```python
from build123d import *

# Parameters (mm, degrees)
SKETCH1_R                = 1.6
SKETCH1_R_2              = 6.45
BOSS_EXTRUDE1_DEPTH      = 3.175
SKETCH4_R                = 1.675
BOSS_EXTRUDE3_DEPTH      = 6.25
SKETCH4_2_R              = 1.675
CUT_EXTRUDE2_DEPTH       = 2.63125
FILLET1_R                = 2
FILLET2_R                = 2
FILLET3_R                = 2
CIRPATTERN2_COUNT        = 3
FILLET1_OF_CIRPATTERN2_R = 2
FILLET2_OF_CIRPATTERN2_R = 2
FILLET3_OF_CIRPATTERN2_R = 2
FILLET5_R                = 0.75


with BuildPart() as part:
    # Sketch1 → Boss-Extrude1 (new body)
    with BuildSketch(Plane.XY):
        with BuildLine():
            Line((15.347308801, 31.210973101), (8.051491314, 33.998880179))
            ThreePointArc((8.051491314, 33.998880179), (5.696175566, 34.15336703), (3.663829908, 32.952971436))
            Line((3.663829908, 32.952971436), (-1.653149933, 27.103867562))
            ThreePointArc((-1.653149933, 27.103867562), (-2.154824203, 26.417727613), (-2.500196213, 25.641078866))
            Line((-2.500196213, 25.641078866), (-9.325438013, 4.478720632))
            ThreePointArc((-9.325438013, 4.478720632), (-9.502063256, 3.613546149), (-9.484560317, 2.730700176))
            Line((-9.484560317, 2.730700176), (-8.507421128, -4.718687488))
            ThreePointArc((-8.507421128, -4.718687488), (-7.54564448, -6.839386894), (-5.565731281, -8.065080174))
            Line((-5.565731281, -8.065080174), (2.031002829, -10.077591551))
            ThreePointArc((2.031002829, -10.077591551), (2.960636861, -10.209852347), (3.895489669, -10.121746843))
            Line((3.895489669, -10.121746843), (25.485057009, -5.483666514))
            ThreePointArc((25.485057009, -5.483666514), (26.373611638, -5.180049941), (27.166902489, -4.677653705))
            Line((27.166902489, -4.677653705), (33.329625608, 0.328323939))
            ThreePointArc((33.329625608, 0.328323939), (34.614533997, 2.205289229), (34.668387555, 4.479291881))
            Line((34.668387555, 4.479291881), (32.591741985, 12.142614371))
            ThreePointArc((32.591741985, 12.142614371), (32.241466178, 13.013831458), (31.697738169, 13.779384986))
            Line((31.697738169, 13.779384986), (16.88625911, 30.157458595))
            ThreePointArc((16.88625911, 30.157458595), (16.17904213, 30.77516119), (15.347308801, 31.210973101))
        make_face()
        with Locations((24.879793107, 5.344918551)):
            Circle(SKETCH1_R, mode=Mode.SUBTRACT)
        with Locations((7.811061307, 24.218992148)):
            Circle(SKETCH1_R, mode=Mode.SUBTRACT)
        Circle(SKETCH1_R, mode=Mode.SUBTRACT)
        with Locations((10.896951472, 9.8546369)):
            Circle(SKETCH1_R_2, mode=Mode.SUBTRACT)
    extrude(amount=BOSS_EXTRUDE1_DEPTH)

    # Sketch4 → Boss-Extrude3 (add, symmetric)
    with BuildSketch(Plane(origin=(0.449621982, -0.475334512, 0), x_dir=(-0.726482741, -0.687184711, 0), z_dir=(0.687184711, -0.726482741, 0))):
        Polygon((-31.72132028, 0), (-31.72132028, -3.175), (-25.539496086, -3.175), (-31.72132028, -5.425), (-41.88132028, -5.425), (-41.88132028, 0), align=None)
        with Locations((-36.80132028, -2.7125)):
            Circle(SKETCH4_R, mode=Mode.SUBTRACT)
    boss_extrude3 = extrude(amount=BOSS_EXTRUDE3_DEPTH, both=True)

    # Sketch4<2> → Cut-Extrude2 (cut, symmetric)
    with BuildSketch(Plane(origin=(0.449621982, -0.475334512, 0), x_dir=(-0.726482741, -0.687184711, 0), z_dir=(0.687184711, -0.726482741, 0))):
        Polygon((-31.72132028, 0), (-31.72132028, -3.175), (-25.539496086, -3.175), (-31.72132028, -5.425), (-41.88132028, -5.425), (-41.88132028, 0), align=None)
        with Locations((-36.80132028, -2.7125)):
            Circle(SKETCH4_2_R, mode=Mode.SUBTRACT)
    cut_extrude2 = extrude(amount=CUT_EXTRUDE2_DEPTH, both=True, mode=Mode.SUBTRACT)

    # Fillet1
    fillet1_edges = [part.edges().sort_by_distance(p)[0] for p in [
        (19.440964609, 21.110601986, 3.175),
        (23.057274153, 17.287486564, 3.175),
        (25.865326768, 14.96244967, 3.175),
        (17.377217607, 24.139682361, 3.175),
        (22.0551547, 13.848979318, 3.175),
        (15.952095481, 20.301054157, 3.175),
    ]]
    fillet(fillet1_edges, radius=FILLET1_R)

    # Fillet2
    fillet2_edges = [part.edges().sort_by_distance(p)[0] for p in [
        (25.302768444, 19.411514101, 1.5875),
        (21.6864589, 23.234629523, 1.5875),
    ]]
    fillet(fillet2_edges, radius=FILLET2_R)

    # Fillet3
    fillet3_edges = [part.edges().sort_by_distance(p)[0] for p in [
        (27.824148706, 31.530905901, 0),
        (33.927207925, 25.078831062, 0),
        (33.927207925, 25.078831062, 5.425),
        (27.824148706, 31.530905901, 5.425),
    ]]
    fillet(fillet3_edges, radius=FILLET3_R)

    # CirPattern2: Boss-Extrude3, Cut-Extrude2 ×3 about axis
    cirpattern2_axis = Axis((10.896951472, 9.8546369, 0), (0, 0, 1))
    for i in range(1, CIRPATTERN2_COUNT):
        add(boss_extrude3.rotate(cirpattern2_axis, i * 360 / CIRPATTERN2_COUNT))
        add(cut_extrude2.rotate(cirpattern2_axis, i * 360 / CIRPATTERN2_COUNT), mode=Mode.SUBTRACT)

    # Fillet1 of CirPattern2
    fillet1_of_cirpattern2_edges = [part.edges().sort_by_distance(p)[0] for p in [
        (-3.123006806, 11.625986784, 3.175),
        (-1.620246501, 16.669360428, 3.175),
        (-1.010731793, 20.263723774, 3.175),
        (-4.71439386, 8.324189266, 3.175),
        (1.858647852, 17.520753147, 3.175),
        (-0.677483256, 9.009311403, 3.175),
        (16.372896612, -3.172678071, 3.175),
        (11.253826762, -4.392936293, 3.175),
        (7.836259441, -5.662262745, 3.175),
        (20.028030667, -2.899960928, 3.175),
        (8.777051863, -1.805821766, 3.175),
        (17.41624219, 0.253545139, 3.175),
    ]]
    fillet(fillet1_of_cirpattern2_edges, radius=FILLET1_OF_CIRPATTERN2_R)

    # Fillet2 of CirPattern2
    fillet2_of_cirpattern2_edges = [part.edges().sort_by_distance(p)[0] for p in [
        (-4.582455452, 17.552001759, 1.5875),
        (-6.085215757, 12.508628115, 1.5875),
        (11.970541423, -7.399605162, 1.5875),
        (17.089611272, -6.17934694, 1.5875),
    ]]
    fillet(fillet2_of_cirpattern2_edges, radius=FILLET2_OF_CIRPATTERN2_R)

    # Fillet3 of CirPattern2
    fillet3_of_cirpattern2_edges = [part.edges().sort_by_distance(p)[0] for p in [
        (-16.33884676, 13.675885219, 0),
        (-13.802715652, 22.187326963, 0),
        (-13.802715652, 22.187326963, 5.425),
        (-16.33884676, 13.675885219, 5.425),
        (21.205552469, -15.642880421, 0),
        (12.566362141, -17.702247326, 0),
        (12.566362141, -17.702247326, 5.425),
        (21.205552469, -15.642880421, 5.425),
    ]]
    fillet(fillet3_of_cirpattern2_edges, radius=FILLET3_OF_CIRPATTERN2_R)

    # Fillet5
    fillet5_edges = [part.edges().sort_by_distance(p)[0] for p in [
        (-7.789671487, 9.240521362, 1.5875),
        (-3.951849266, 21.140080535, 1.5875),
        (20.879758905, -6.473021336, 1.5875),
        (8.655527257, -9.099149384, 1.5875),
        (20.045714571, 26.663830856, 2.5875),
        (28.432123998, 17.390399731, 2.5875),
    ]]
    fillet(fillet5_edges, radius=FILLET5_R)


solid = part.part
```
The listing builds one solid part. Answer for the finished solid, in the listing's coordinates (mm). A direction names the side the tool comes from. Round coordinates to 2 decimals unless told otherwise and drop trailing zeros. Use one line per item in the form item = value. Start each with the question number.
1. Given pin 1 Ø3 at (x, y) = (8, -12) entering from +Z (3 decimals); pin 2 Ø4 at (x, y) = (0, 0) entering from +Z (3 decimals); pin 3 Ø2 at (x, z) = (-5, 4.5) entering from -Y; pin 4 Ø3 at (x, z) = (0, 1.5) entering from -Y, each flat-ended and moving along its own axis, determine where each tip first touches the part or whether it passes through.
2. For a pull along X with two mould halves and no side action, classify faces 6 (the face through (23.53, -5.904, 1.775)), 7 (the face through (10.06, 16.25, 1.57)), 8 (the face through (11, -12, 5.425)) as pulls with the +X half, pulls with the -X half, needs draft (parallel to the pull), parting line crosses it, or undercut.
3. Consider line 1 (Z direction, x = 1.5, y = 15) (3 decimals); line 2 (X direction, y = 8.5, z = 2.7); line 3 (X direction, y = 25, z = 2.7). Determine where each line is inside the solid, lowest interval first. Write a range as [from, to].
4. A tool of negligible diameter and unlimited length cuts with its end or side. For faces 1 (the face through (17.5, 0.3, 3.2)), 2 (the face through (-1.6, 21.31, 3.55)), 3 (the face through (-0.683, 8.955, 3.205)), 4 (the face through (-2.59, 16.09, 3.55)), 5 (the face through (-8.666, 6.523, 1.775)), from which of +Z, -Z, +X, -X, +Y, -Y can it reach the whole face along a straight path? Write none if from no direction.
Geometry check:
q1.pin_1 = 5.425
q1.pin_2 = 3.175
q1.pin_3 = 7.43
q1.pin_4 = -9.94
q2.face_6 = pulls with the +X half
q2.face_7 = undercut
q2.face_8 = needs draft
q3.line_1 = [0, 3.175]
q3.line_2 = [-8.03, 4.59], [17.2, 33.58]
q3.line_3 = [-2.71, 6.41], [9.21, 23.55], [31.21, 34]
q4.face_1 = +Z, -X
q4.face_2 = +Z, +Y
q4.face_3 = +Z, -Y
q4.face_4 = +Z
q4.face_5 = +Z, -Z, -X
